Study the drawing (mm; zero at the part's minimum x, y, z) and answer. A direction names the side the tool comes from. Round coordinates to 2 decimals unless told otherwise and drop trailing zeros. Order: outer loops, then holes, each group sorted by start corner. A loop starts at its lowest first (then second) coordinate and runs counter-clockwise, first axis right, second up. Notation, with made-up numbers: (49.5, 35) - (89.5, 35) arc R16 cw to (89.5, 66) - close; hole circle Ø11 at (18.25, -4.75). An arc over 180 degrees is marked (long way). Put each result on its own line as item: value. Start each with the question number.
Q1. Section D-D on x = 11.5 is taken. Give the vertices of the cut face in (y, z), then the cut area to 3 significant figures.
Q2. Section B-B on x = 4.5 is taken. Give the vertices of the cut face in (y, z), then the cut area to 3 significant figures.
Q3. Which of the six approach directions +Z, -Z, +X, -X, +Y, -Y give full straight-line access (tool end or side, diameter ignored) to the marked faces 1, 2, 3, 4 and 5?
Q4. Find the intervals of material crossed by line 1 along X through (y, z) = (3, 24); line 2 along Z through (x, y) = (12.75, 10.5); line 3 along Z through (x, y) = (10.25, 14.25), in increasing order. Write a range as from..to.
Q5. Section A-A on z = 3.75 is taken. Give the vertices of the cut face in (x, y).
Q6. Section C-C on y = 6.5 is taken. Give the vertices of the cut face in (x, z), then the cut area to 3 significant figures.
Q7. For a pull along Z with two mould halves and no side action, classify the marked faces 6, 7, 8 and 9 as pulls with the +Z half, pulls with the -Z half, needs draft (parallel to the pull), parting line crosses it, or undercut.
Q8. Each of these flat-tipped pins is pushed along its axis until it touches: pin 1 Ø1.5 at (x, z) = (14, 5) entering from -Y; pin 2 Ø0.8 at (y, z) = (17, 14.5) entering from +X; pin 3 Ø3 at (x, z) = (14, 20.5) entering from +Y; pin 4 Ø4.5 at (x, z) = (4, 24.5) entering from +Y. Where does it stop, or does it pass through?
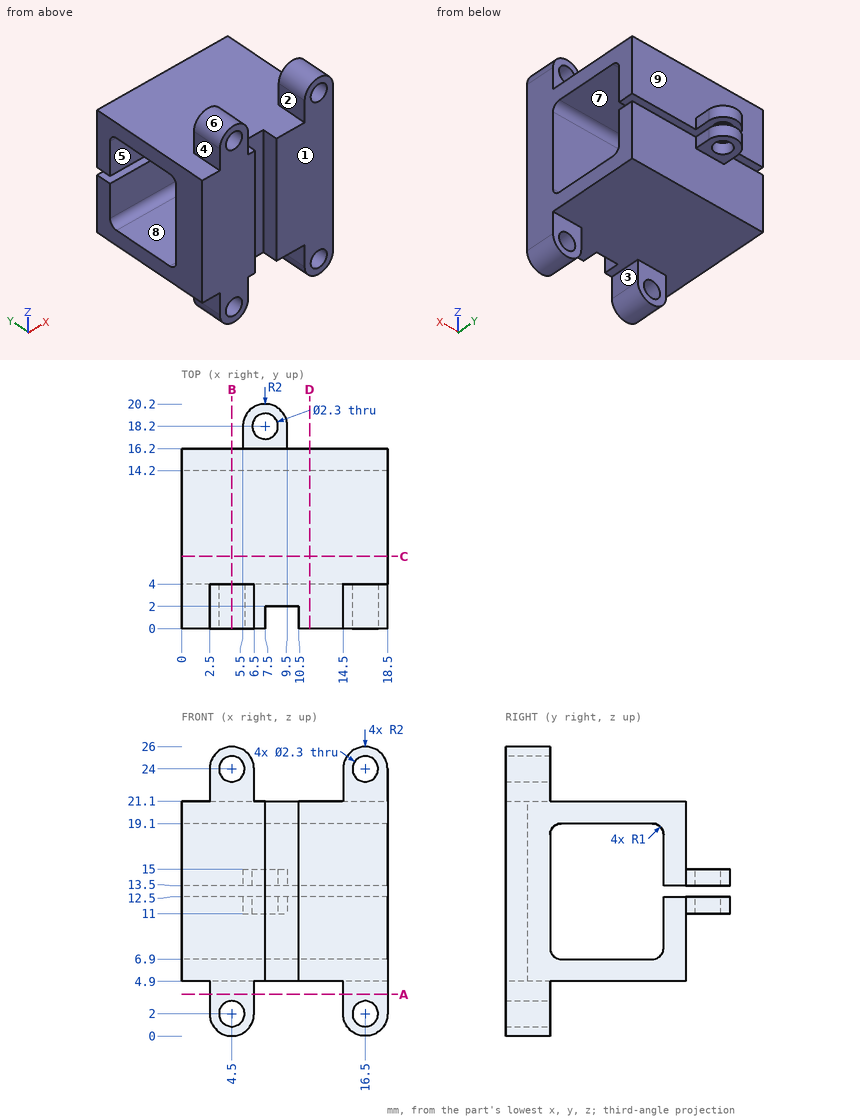
Findings:
1. outline: (0, 4.9) - (16.2, 4.9) - (16.2, 12.5) - (14.2, 12.5) - (14.2, 7.9) arc R1 cw to (13.2, 6.9) - (5, 6.9) arc R1 cw to (4, 7.9) - (4, 18.1) arc R1 cw to (5, 19.1) - (13.2, 19.1) arc R1 cw to (14.2, 18.1) - (14.2, 13.5) - (16.2, 13.5) - (16.2, 21.1) - (0, 21.1) - close
1. area: 137 mm2
2. outline: (0, 0) - (4, 0) - (4, 0.85) - (0, 0.85) - close; (0, 3.15) - (4, 3.15) - (4, 4.9) - (16.2, 4.9) - (16.2, 12.5) - (14.2, 12.5) - (14.2, 7.9) arc R1 cw to (13.2, 6.9) - (5, 6.9) arc R1 cw to (4, 7.9) - (4, 18.1) arc R1 cw to (5, 19.1) - (13.2, 19.1) arc R1 cw to (14.2, 18.1) - (14.2, 13.5) - (16.2, 13.5) - (16.2, 21.1) - (4, 21.1) - (4, 22.85) - (0, 22.85) - close; (0, 25.15) - (4, 25.15) - (4, 26) - (0, 26) - close
2. area: 158 mm2
3. face 1: +Z, -Z, +X, -X, -Y
3. face 2: +Z, +Y, -Y
3. face 3: -Z, +Y, -Y
3. face 4: +Z, -X, +Y, -Y
3. face 5: +X, -X
4. line 1: 2.5..3.35, 5.65..6.5, 14.5..15.35, 17.65..18.5
4. line 2: 4.9..6.9, 19.1..21.1
4. line 3: 4.9..12.5, 13.5..21.1
5. outline: (2.5, 0) - (6.5, 0) - (6.5, 4) - (2.5, 4) - close; (14.5, 0) - (18.5, 0) - (18.5, 4) - (14.5, 4) - close
6. outline: (0, 4.9) - (18.5, 4.9) - (18.5, 6.9) - (0, 6.9) - close; (0, 19.1) - (18.5, 19.1) - (18.5, 21.1) - (0, 21.1) - close
6. area: 74.0 mm2
7. face 6: pulls with the +Z half
7. face 7: undercut
7. face 8: undercut
7. face 9: needs draft
8. pin 1: y = 0
8. pin 2: x = 9.5
8. pin 3: y = 16.2
8. pin 4: y = 4
